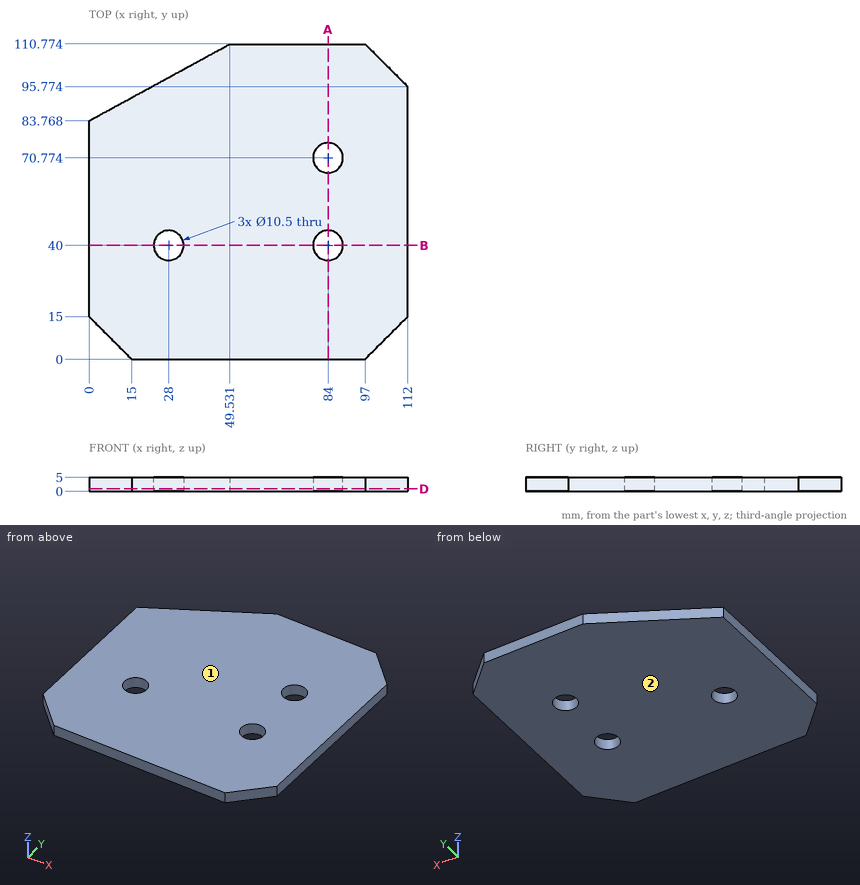
Part print with two shaded views. Sizes in mm from the minimum x, y, z corner. Give positions to 0.01 mm unless a question says otherwise; leave off trailing zeros. Order: outer loops, then holes, each group sorted by start corner. A loop starts at its lowest first (then second) coordinate and runs counter-clockwise, first axis right, second up. Notation, with made-up numbers: (38, 29) - (75, 29) arc R21 ccw to (75, 51) - close; hole circle Ø2 at (-38.5, 65.5). An arc over 180 degrees is marked (long way). Write each question's results on one line, items separated by ' | '.
1. Probe L1, parallel to Y at x = 84, z = 2.3; L2, parallel to X at y = 72.5, z = 1.95; L3, parallel to X at y = 75, z = 2.75 (1 decimal). List the from-to ranges inside material, lowest first. Write a range as from..to.
Calculated:
L1: y = 0..34.75, 45.25..65.52, 76.02..110.77 | L2: x = 0..79.04, 88.96..112 | L3: x = 0..80.9, 87.1..112
2. Pull direction Z, two halves, no side cores. Call the marked faces 1 and 2: released by +Z, released by -Z, zero draft, split by the parting line, or undercut.
Calculated:
face 1: released by +Z | face 2: released by -Z
3. Saw through at B-B on y = 40. List the corners of the cut face in (x, z).
Calculated:
outline: (0, 0) - (22.75, 0) - (22.75, 5) - (0, 5) - close; (33.25, 0) - (78.75, 0) - (78.75, 5) - (33.25, 5) - close; (89.25, 0) - (112, 0) - (112, 5) - (89.25, 5) - close
4. Saw through at A-A on x = 84. List the corners of the cut face in (y, z).
Calculated:
outline: (0, 0) - (34.75, 0) - (34.75, 5) - (0, 5) - close; (45.25, 0) - (65.52, 0) - (65.52, 5) - (45.25, 5) - close; (76.02, 0) - (110.77, 0) - (110.77, 5) - (76.02, 5) - close
5. Saw through at D-D on z = 0.95. List the corners of the cut face in (x, y).
Calculated:
outline: (0, 15) - (15, 0) - (97, 0) - (112, 15) - (112, 95.77) - (97, 110.77) - (49.53, 110.77) - (0, 83.77) - close; hole circle Ø10.5 at (28, 40); hole circle Ø10.5 at (84, 40); hole circle Ø10.5 at (84, 70.77)
6. Pin check, flat tips, straight feed: pin 1 (10 mm diameter, centred on x = 95.5, y = 21.5, fed in from -Z); pin 2 (9.5 mm diameter, centred on x = 28, y = 40, fed in from +Z). Stop position of each tip, or through.
Calculated:
pin 1: stops at z = 0 | pin 2: passes through
